Here's the drawing with two shaded views (mm, measured from the low corner). I have some questions. Give positions to 0.01 mm unless a question says otherwise; leave off trailing zeros. Write each loop counter-clockwise with the first axis right and the second up, starting at its lowest first coordinate (ties: lowest second). Pieces come first, ordered by that corner, then holes. Notation, with made-up numbers: (-2.75, 49.5) -> (34.25, 49.5) arc R26 cw to (34.25, 64.5) -> close; hole circle Ø1 at (-12.5, 86). An arc over 180 degrees is marked (long way). Put each result on its own line as item: value. Start each with the question number.
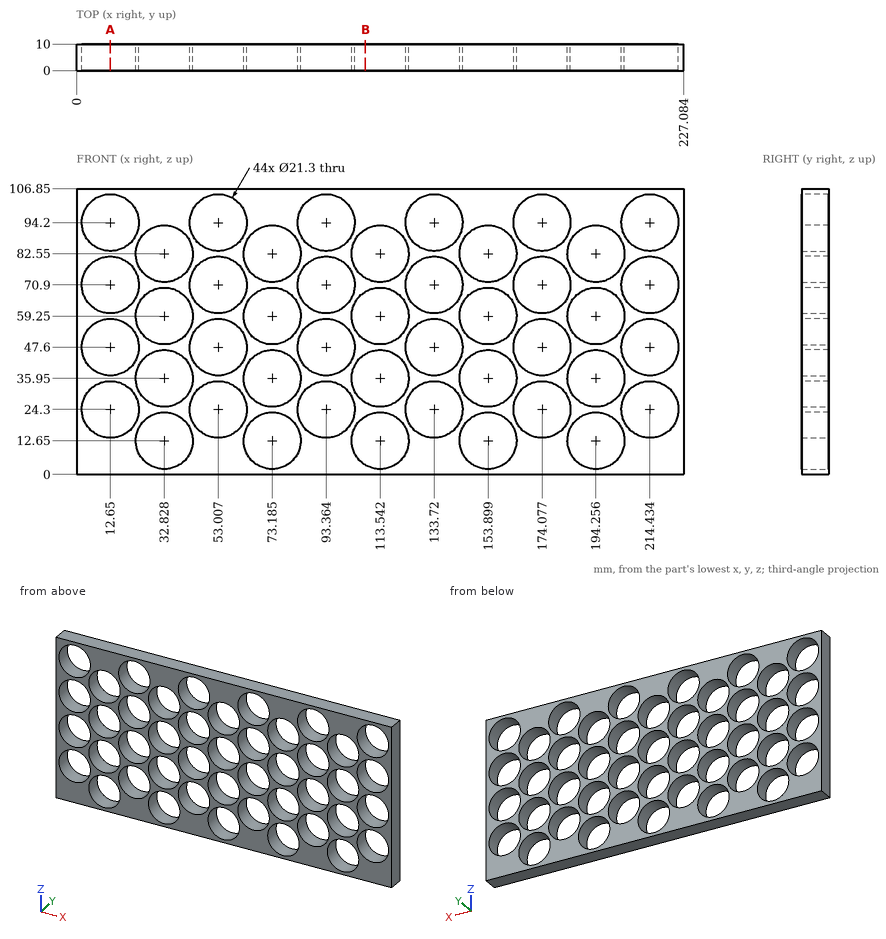
1) I want a section at B-B, the plane x = 108. State how many separate pieces and enclosed holes the cut face has, and give its area (3 significant figures).
2) I'm going to push a flat-ended pin straight in: pin 1 Ø24.5 at (x, z) = (93.36, 47.6) entering from +Y. Where does the tip first touch, or does it pass through?
3) I need wall thicknesses on probe 1 along X at (y, z) = (5, 12.65) (1 decimal); probe 2 along X at (y, z) = (6.5, 59.5) (1 decimal); probe 3 along Z at (x, y) = (36, 6). Which ranges of each line are inside material? Lowest first, please.
4) I want a section at A-A, the plane x = 12.65. Write out the boundary of the cut face in (y, z).
Established:
1. separate pieces: 5
1. enclosed holes: 0
1. area: 341 mm2
2. pin 1: stops at y = 10
3. probe 1: x = 0 to 22.2, 43.5 to 62.5, 83.8 to 102.9, 124.2 to 143.2, 164.5 to 183.6, 204.9 to 227.1
3. probe 2: x = 0 to 22.2, 43.5 to 62.5, 83.8 to 102.9, 124.2 to 143.3, 164.5 to 183.6, 204.9 to 227.1
3. probe 3: z = 0 to 2.48, 22.82 to 25.78, 46.12 to 49.08, 69.42 to 72.38, 92.72 to 106.85
4. outline: (0, 0) -> (10, 0) -> (10, 13.65) -> (0, 13.65) -> close; (0, 34.95) -> (10, 34.95) -> (10, 36.95) -> (0, 36.95) -> close; (0, 58.25) -> (10, 58.25) -> (10, 60.25) -> (0, 60.25) -> close; (0, 81.55) -> (10, 81.55) -> (10, 83.55) -> (0, 83.55) -> close; (0, 104.85) -> (10, 104.85) -> (10, 106.85) -> (0, 106.85) -> close
